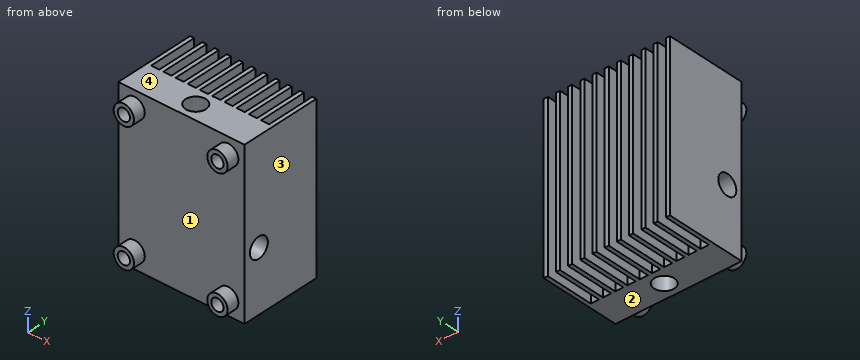
```python
from build123d import *

# Parameters (mm, degrees)
EXTRUDE1_DEPTH       = 40
SKETCH2_R            = 2.5
EXTRUDE2_DEPTH       = 48.331279298
SKETCH3_R            = 2.5
EXTRUDE3_DEPTH       = 55.415071442
SKETCH4_R            = 2.5
SKETCH4_R_2          = 1.5
EXTRUDE4_DEPTH       = 3
LPATTERN6_COUNT      = 2
LPATTERN6_PITCH      = 23
LPATTERN6_COUNT_DIR2 = 2
LPATTERN6_PITCH_DIR2 = 32


with BuildPart() as part:
    # Sketch1 → Extrude1 (new body)
    with BuildSketch(Plane.XY):
        Polygon((-15.5, 0), (-15.5, 20), (-14.5, 20), (-14.5, 8), (-12.5, 8), (-12.5, 20), (-11.5, 20), (-11.5, 8), (-9.5, 8), (-9.5, 20), (-8.5, 20), (-8.5, 8), (-6.5, 8), (-6.5, 20), (-5.5, 20), (-5.5, 8), (-3.5, 8), (-3.5, 20), (-2.5, 20), (-2.5, 8), (-0.5, 8), (-0.5, 20), (0.5, 20), (0.5, 8), (2.5, 8), (2.5, 20), (3.5, 20), (3.5, 8), (5.5, 8), (5.5, 20), (6.5, 20), (6.5, 8), (8.5, 8), (8.5, 20), (9.5, 20), (9.5, 8), (11.5, 8), (11.5, 20), (12.5, 20), (12.5, 8), (14.5, 8), (14.5, 20), (15.5, 20), (15.5, 0), align=None)
    extrude(amount=-EXTRUDE1_DEPTH)

    # Sketch2 → Extrude2 (cut, through all)
    with BuildSketch(Plane.XY):
        with Locations((0, 4)):
            Circle(SKETCH2_R)
    extrude(amount=-EXTRUDE2_DEPTH, mode=Mode.SUBTRACT)

    # Sketch3 → Extrude3 (cut, through all)
    with BuildSketch(Plane(origin=(15.5, 0, 0), x_dir=(0, 0, -1), z_dir=(1, 0, 0))):
        with Locations(Location((25, 4, 0), (0, 0, 90))):
            Circle(SKETCH3_R)
    extrude(amount=-EXTRUDE3_DEPTH, mode=Mode.SUBTRACT)

    # Sketch4 → Extrude4 (add)
    with BuildSketch(Plane.XZ):
        with Locations((11.5, -4)):
            Circle(SKETCH4_R)
        with Locations((11.5, -4)):
            Circle(SKETCH4_R_2, mode=Mode.SUBTRACT)
    extrude4 = extrude(amount=EXTRUDE4_DEPTH)

    # LPattern6: Extrude4 2 × 2
    with Locations(*[(-i * LPATTERN6_PITCH, 0, -j * LPATTERN6_PITCH_DIR2) for i in range(LPATTERN6_COUNT) for j in range(LPATTERN6_COUNT_DIR2) if (i, j) != (0, 0)]):
        add(extrude4)


solid = part.part
```
Model file for the job. Use its own axes, mm. Face numbers are marked on the shaded views. Round coordinates to 2 decimals unless told otherwise and drop trailing zeros. Write each loop counter-clockwise with the first axis right and the second up, starting at its lowest first coordinate (ties: lowest second). Pieces come first, ordered by that corner, then holes. Notation, with made-up numbers: (81.5, 24.5) - (85.5, 24.5) arc R15 ccw to (85.5, 34.5) - close; hole circle Ø5 at (51.25, -16). An arc over 180 degrees is marked (long way). One line per item, written item: value.
(1) Cut at C-C, the plane y = 17. Give the number of separate pieces and of enclosed holes in the cut face, plus the area to 3 significant figures.
Values follow:
separate pieces: 11
enclosed holes: 0
area: 440 mm²
(2) Cut at A-A, the plane y = 2.5. Give the cut face in (x, z).
Values follow:
outline: (-15.5, -40) - (-2, -40) - (-2, -27) - (-15.5, -27) - close; (-15.5, -23) - (-2, -23) - (-2, 0) - (-15.5, 0) - close; (2, -40) - (15.5, -40) - (15.5, -27) - (2, -27) - close; (2, -23) - (15.5, -23) - (15.5, 0) - (2, 0) - close
(3) Cut at B-B, the plane x = -1. Give the cut face in (y, z).
Values follow:
outline: (0, -40) - (1.71, -40) - (1.71, -26) arc R2.5 cw to (1.71, -24) - (1.71, 0) - (0, 0) - close; (6.29, -40) - (8, -40) - (8, 0) - (6.29, 0) - (6.29, -24) arc R2.5 cw to (6.29, -26) - close
(4) Drop a flat-ended pin along its axis: P1, Ø0.6, axis at x = 13, z = -29.5, coming from the +Y side. Give the stop position or say it passes through.
Values follow:
P1: stops at y = 8
(5) Two-plate mould, pull along Z, no slides. Class the marked faces 1, 2, 3 and 4: pulls with the +Z half, pulls with the -Z half, needs draft (parallel to the pull), parting line crosses it, or undercut.
Values follow:
face 1: undercut
face 2: pulls with the -Z half
face 3: needs draft
face 4: pulls with the +Z half
(6) Wall check: probe 1 along Z at (x, y) = (-11.5, -0.6); probe 2 along Z at (x, y) = (10, 4); probe 3 along X at (y, z) = (4, -30.5). Give the ranges that are in metal, low to high.
Values follow:
probe 1: z = -38.5 to -37.5, -34.5 to -33.5, -6.5 to -5.5, -2.5 to -1.5
probe 2: z = -40 to -27.5, -22.5 to 0
probe 3: x = -15.5 to -2.5, 2.5 to 15.5
